```python
from build123d import *

# Parameters (mm, degrees)
SKETCH3_R                = 43.942
BOSS_EXTRUDE1_DEPTH      = 15.24
BOSS_EXTRUDE2_REACH      = 2156.162
BOSS_EXTRUDE2_END_RADIUS = 78.322932
SKETCH4_W                = 3.175
SKETCH4_H                = 203.2
CUT_EXTRUDE1_REACH       = 2145.535
FILLET1_R                = 2.54
CIRPATTERN1_COUNT        = 4
FILLET1_OF_CIRPATTERN1_R = 2.54


with BuildPart() as part:
    # Sketch2 → Revolve1 (revolve)
    with BuildSketch(Plane(origin=(0, 0, 0), x_dir=(0, 0, -1), z_dir=(1, 0, 0)), mode=Mode.PRIVATE) as revolve1_sk:
        with BuildLine():
            Line((76.2, 78.322932), (2111.6925, 78.322932))
            Line((2111.6925, 78.322932), (2111.6925, 0))
            Line((2111.6925, 0), (0, 0))
            add(Edge.make_bspline(
                [(0, 0), (0.00157185, 0.031106382), (0.00598179, 0.093218427), (0.019741162, 0.217041654), (0.056245749, 0.471623897), (0.120220676, 0.824555102), (0.289900607, 1.607620967), (0.681695021, 3.044497502), (1.369417811, 5.088592926), (2.663624448, 8.328390532), (4.627219491, 12.504828431), (7.221628503, 17.313832891), (10.478488809, 22.663697626), (14.048468312, 27.97193092), (17.830107282, 33.131203754), (21.803068789, 38.144384751), (25.954684106, 43.010577273), (30.277267993, 47.72553477), (34.76726888, 52.281456881), (39.424593478, 56.666373482), (44.252629149, 60.862995207), (49.25851273, 64.846416869), (54.379271658, 68.526766678), (59.025760285, 71.483086359), (63.137367168, 73.775059871), (66.620488281, 75.459145189), (69.291079417, 76.576884505), (71.652609302, 77.398960624), (73.545502358, 77.917349185), (74.790486934, 78.170322816), (75.589714748, 78.281706661), (75.99027716, 78.31490275), (76.130043485, 78.321823203), (76.2, 78.322932)],
                knots=[0, 0, 0, 0, 0, 0.00110147, 0.00220294, 0.004405879, 0.009096351, 0.013786822, 0.030539543, 0.057061285, 0.08533897, 0.137140357, 0.193696574, 0.250252697, 0.306809175, 0.363365414, 0.419921856, 0.476478205, 0.533034532, 0.589590952, 0.646147292, 0.702703654, 0.75926004, 0.815816409, 0.86911958, 0.89739782, 0.925675959, 0.952619519, 0.971471661, 0.985785918, 0.995050665, 0.997525332, 1, 1, 1, 1, 1], degree=4))
        make_face()
    revolve(revolve1_sk.sketch.rotate(Axis((0, 0, -2111.6925), (0, 0, 1)), 90), axis=Axis((0, 0, -2111.6925), (0, 0, 1)))

    # Sketch3 → Boss-Extrude1 (add)
    with BuildSketch(Plane(origin=(0, 0, -2111.6925), x_dir=(-1, 0, 0), z_dir=(0, 0, -1))):
        with Locations(Location((0, 0, 0), (0, 0, 270))):
            Circle(SKETCH3_R)
    extrude(amount=BOSS_EXTRUDE1_DEPTH)

    # Boss-Extrude2: up to this cylinder (the profile starts outside it)
    boss_extrude2_end = Plane(origin=(0, 0, -2006.9175), z_dir=(0, 0, -1)) * Cylinder(BOSS_EXTRUDE2_END_RADIUS, 4469.969864, mode=Mode.PRIVATE)
    # Sketch4 → Boss-Extrude2 (add, up to the surface)
    with BuildSketch(Plane(origin=(0, 254, 0), x_dir=(1, 0, 0), z_dir=(0, 1, 0)), mode=Mode.PRIVATE) as boss_extrude2_sk1:
        with Locations((0, 2006.9175)):
            Rectangle(SKETCH4_W, SKETCH4_H)
    boss_extrude2_tool1 = extrude(boss_extrude2_sk1.sketch, amount=-BOSS_EXTRUDE2_REACH, mode=Mode.PRIVATE) - boss_extrude2_end
    boss_extrude2 = boss_extrude2_tool1.solids().sort_by_distance((0, 254, -2006.9175))[0]
    add(boss_extrude2)

    # Sketch5 → Cut-Extrude1 (cut, up to next)
    with BuildSketch(Plane.ZY.offset(1.5875), mode=Mode.PRIVATE) as cut_extrude1_sk1:
        Polygon((-2108.5175, 224.356842107), (-2006.9175, 224.356842107), (-1905.3175, 78.306842107), (-1905.3175, 254), (-2108.5175, 254), align=None)
    cut_extrude1_tool1 = extrude(cut_extrude1_sk1.sketch, amount=-CUT_EXTRUDE1_REACH, mode=Mode.PRIVATE) & part.part
    cut_extrude1 = cut_extrude1_tool1.solids().sort_by_distance((-1.5875, 204.128915, -1969.534252))[0]
    add(cut_extrude1, mode=Mode.SUBTRACT)

    # Fillet1
    # the kernel refuses this fillet: 2.54 mm, written as the material it adds along each edge
    with BuildSketch(Plane(origin=(-1.5875, 78.306842107, -1899.190797857), x_dir=(-0.9993639751499004, -0.03566013422001241, 0), z_dir=(0, 0, -1))) as fillet1_piece_1_section:
        with BuildLine():
            CenterArc((2.450992889, 2.539698904), FILLET1_R, 182.043608468, 87.074170625)
            Line((-0.087391608, 2.449122163), (0, 0))
            ThreePointArc((0, 0), (1.205942189, 0.009284527), (2.411884379, 0))
        make_face()
    fillet1_piece_1 = extrude(amount=209.326702143, mode=Mode.PRIVATE)
    fillet1_piece_1 = split(fillet1_piece_1, bisect_by=Plane(origin=(-3.095055571, 78.248638535, -1905.277010558), z_dir=(0, -0.5710644881985995, -0.8209052017854874)), keep=Keep.TOP, mode=Mode.PRIVATE)
    add(fillet1_piece_1)
    with BuildSketch(Plane(origin=(1.5875, 78.306842107, -1899.190797857), x_dir=(0.9993639751499004, -0.035660134220013434, 0), z_dir=(0, 0, -1))) as fillet1_piece_2_section:
        with BuildLine():
            CenterArc((2.450992889, -2.539698904), FILLET1_R, 90.882220907, 87.074170625)
            Line((-0.087391608, -2.449122163), (0, 0))
            ThreePointArc((0, 0), (1.205942189, -0.009284527), (2.411884379, 0))
        make_face()
    fillet1_piece_2 = extrude(amount=209.326702143, mode=Mode.PRIVATE)
    fillet1_piece_2 = split(fillet1_piece_2, bisect_by=Plane(origin=(3.095055571, 78.248638535, -1905.277010558), z_dir=(0, -0.5710644881985995, -0.8209052017854874)), keep=Keep.TOP, mode=Mode.PRIVATE)
    add(fillet1_piece_2)

    # CirPattern1: Boss-Extrude2, Cut-Extrude1 ×4 about axis
    cirpattern1_axis = Axis((0, 0, 0), (0, 0, 1))
    add([boss_extrude2.rotate(cirpattern1_axis, i * 360 / CIRPATTERN1_COUNT) for i in range(1, CIRPATTERN1_COUNT)])
    add([cut_extrude1.rotate(cirpattern1_axis, i * 360 / CIRPATTERN1_COUNT) for i in range(1, CIRPATTERN1_COUNT)], mode=Mode.SUBTRACT)

    # Fillet1 of CirPattern1
    # the kernel refuses this fillet: 2.54 mm, written as the material it adds along each edge
    with BuildSketch(Plane(origin=(-78.306842107, -1.5875, -1899.190797857), x_dir=(0.03566013422001848, -0.9993639751499002, 0), z_dir=(0, 0, -1))) as fillet1_of_cirpattern1_piece_1_section:
        with BuildLine():
            CenterArc((2.450992889, 2.539698904), FILLET1_OF_CIRPATTERN1_R, 182.043608468, 87.074170625)
            Line((-0.087391608, 2.449122163), (0, 0))
            ThreePointArc((0, 0), (1.205942189, 0.009284527), (2.411884379, 0))
        make_face()
    fillet1_of_cirpattern1_piece_1 = extrude(amount=209.326702143, mode=Mode.PRIVATE)
    fillet1_of_cirpattern1_piece_1 = split(fillet1_of_cirpattern1_piece_1, bisect_by=Plane(origin=(-78.248638535, -3.095055571, -1905.277010558), z_dir=(0.5710644881985995, 0, -0.8209052017854874)), keep=Keep.TOP, mode=Mode.PRIVATE)
    add(fillet1_of_cirpattern1_piece_1)
    with BuildSketch(Plane(origin=(-78.306842107, 1.5875, -1899.190797857), x_dir=(0.03566013422001241, 0.9993639751499004, 0), z_dir=(0, 0, -1))) as fillet1_of_cirpattern1_piece_2_section:
        with BuildLine():
            CenterArc((2.450992889, -2.539698904), FILLET1_OF_CIRPATTERN1_R, 90.882220907, 87.074170625)
            Line((-0.087391608, -2.449122163), (0, 0))
            ThreePointArc((0, 0), (1.205942189, -0.009284527), (2.411884379, 0))
        make_face()
    fillet1_of_cirpattern1_piece_2 = extrude(amount=209.326702143, mode=Mode.PRIVATE)
    fillet1_of_cirpattern1_piece_2 = split(fillet1_of_cirpattern1_piece_2, bisect_by=Plane(origin=(-78.248638535, 3.095055571, -1905.277010558), z_dir=(0.5710644881985995, 0, -0.8209052017854874)), keep=Keep.TOP, mode=Mode.PRIVATE)
    add(fillet1_of_cirpattern1_piece_2)
    with BuildSketch(Plane(origin=(1.5875, -78.306842107, -1899.190797857), x_dir=(0.9993639751499002, 0.035660134220018555, 0), z_dir=(0, 0, -1))) as fillet1_of_cirpattern1_piece_3_section:
        with BuildLine():
            CenterArc((2.450992889, 2.539698904), FILLET1_OF_CIRPATTERN1_R, 182.043608468, 87.074170625)
            Line((-0.087391608, 2.449122163), (0, 0))
            ThreePointArc((0, 0), (1.205942189, 0.009284527), (2.411884379, 0))
        make_face()
    fillet1_of_cirpattern1_piece_3 = extrude(amount=209.326702143, mode=Mode.PRIVATE)
    fillet1_of_cirpattern1_piece_3 = split(fillet1_of_cirpattern1_piece_3, bisect_by=Plane(origin=(3.095055571, -78.248638535, -1905.277010558), z_dir=(0, 0.5710644881985995, -0.8209052017854874)), keep=Keep.TOP, mode=Mode.PRIVATE)
    add(fillet1_of_cirpattern1_piece_3)
    with BuildSketch(Plane(origin=(-1.5875, -78.306842107, -1899.190797857), x_dir=(-0.9993639751499004, 0.03566013422001239, 0), z_dir=(0, 0, -1))) as fillet1_of_cirpattern1_piece_4_section:
        with BuildLine():
            CenterArc((2.450992889, -2.539698904), FILLET1_OF_CIRPATTERN1_R, 90.882220907, 87.074170625)
            Line((-0.087391608, -2.449122163), (0, 0))
            ThreePointArc((0, 0), (1.205942189, -0.009284527), (2.411884379, 0))
        make_face()
    fillet1_of_cirpattern1_piece_4 = extrude(amount=209.326702143, mode=Mode.PRIVATE)
    fillet1_of_cirpattern1_piece_4 = split(fillet1_of_cirpattern1_piece_4, bisect_by=Plane(origin=(-3.095055571, -78.248638535, -1905.277010558), z_dir=(0, 0.5710644881985995, -0.8209052017854874)), keep=Keep.TOP, mode=Mode.PRIVATE)
    add(fillet1_of_cirpattern1_piece_4)
    with BuildSketch(Plane(origin=(78.306842107, 1.5875, -1899.190797857), x_dir=(-0.03566013422001829, 0.9993639751499002, 0), z_dir=(0, 0, -1))) as fillet1_of_cirpattern1_piece_5_section:
        with BuildLine():
            CenterArc((2.450992889, 2.539698904), FILLET1_OF_CIRPATTERN1_R, 182.043608468, 87.074170625)
            Line((-0.087391608, 2.449122163), (0, 0))
            ThreePointArc((0, 0), (1.205942189, 0.009284527), (2.411884379, 0))
        make_face()
    fillet1_of_cirpattern1_piece_5 = extrude(amount=209.326702143, mode=Mode.PRIVATE)
    fillet1_of_cirpattern1_piece_5 = split(fillet1_of_cirpattern1_piece_5, bisect_by=Plane(origin=(78.248638535, 3.095055571, -1905.277010558), z_dir=(-0.5710644881985995, 0, -0.8209052017854874)), keep=Keep.TOP, mode=Mode.PRIVATE)
    add(fillet1_of_cirpattern1_piece_5)
    with BuildSketch(Plane(origin=(78.306842107, -1.5875, -1899.190797857), x_dir=(-0.0356601342200124, -0.9993639751499004, 0), z_dir=(0, 0, -1))) as fillet1_of_cirpattern1_piece_6_section:
        with BuildLine():
            CenterArc((2.450992889, -2.539698904), FILLET1_OF_CIRPATTERN1_R, 90.882220907, 87.074170625)
            Line((-0.087391608, -2.449122163), (0, 0))
            ThreePointArc((0, 0), (1.205942189, -0.009284527), (2.411884379, 0))
        make_face()
    fillet1_of_cirpattern1_piece_6 = extrude(amount=209.326702143, mode=Mode.PRIVATE)
    fillet1_of_cirpattern1_piece_6 = split(fillet1_of_cirpattern1_piece_6, bisect_by=Plane(origin=(78.248638535, -3.095055571, -1905.277010558), z_dir=(-0.5710644881985995, 0, -0.8209052017854874)), keep=Keep.TOP, mode=Mode.PRIVATE)
    add(fillet1_of_cirpattern1_piece_6)


solid = part.part
```
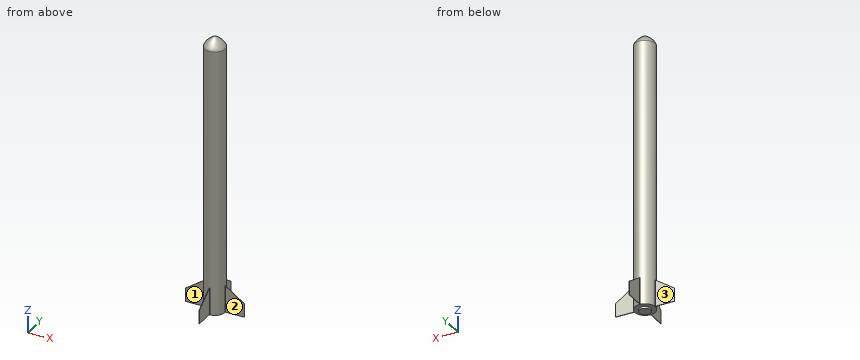
Geometry: final body of the model. Coordinates: model frame, mm. Face numbers are marked on the shaded views. A direction names the side the tool comes from. Round coordinates to 2 decimals unless told otherwise and drop trailing zeros. Write each loop counter-clockwise with the first axis right and the second up, starting at its lowest first coordinate (ties: lowest second). Pieces come first, ordered by that corner, then holes.
Item 1: Set-up query: the marked faces 1, 2 and 3. Return all of +Z, -Z, +X, -X, +Y, -Y with unobstructed straight access to the full face (end or side cutting, diameter ignored); none if empty.
Item 2: Section query A-A (z = -1505). Return loops of the section in (x, y).
Item 3: Section query C-C (x = 153). Return loops of the section in (y, z).
Item 4: Pin query (flat end, axial travel): P1, Ø9, axis at x = 176, y = -0.5, coming from the -Z side; P2, Ø6, axis at y = -60, z = -1503, coming from the -X side; P3, Ø2, axis at y = 56.5, z = -811, coming from the +X side. Return the tip coordinate at first contact, or that it passes through.
Item 5: Material intervals for L1, parallel to X at y = 185.5, z = -2030; L2, parallel to Y at x = -65, z = -1863, sorted ascending.
Item 6: Section query B-B (y = 151). Return loops of the section in (x, z), plus the area to 3 significant figures.
Completed:
1. face 1: +Z, -Z, -X, -Y
1. face 2: +Z, -Z, +X, -Y
1. face 3: +Z, -Z, -X, +Y
2. outline: circle Ø156.65 at (0, 0)
3. outline: (-1.59, -2108.52) - (1.59, -2108.52) - (1.59, -1957.28) - (-1.59, -1957.28) - close
4. P1: stops at z = -2108.52
4. P2: stops at x = -53.72
4. P3: stops at x = 55.27
5. L1: x = -1.59 to 1.59
5. L2: y = -43.7 to 43.7
6. outline: (-1.59, -2108.52) - (1.59, -2108.52) - (1.59, -1955.89) - (-1.59, -1955.89) - close
6. area: 485 mm2
